The listing builds one solid part. Answer for the finished solid, in the listing's coordinates (mm). A direction names the side the tool comes from. Round coordinates to 2 decimals unless told otherwise and drop trailing zeros. Write each loop counter-clockwise with the first axis right and the second up, starting at its lowest first coordinate (ties: lowest second). Pieces come first, ordered by that corner, then holes.
(1) A cutting plane is placed at C-C, the plane y = 3.25. Give the vertices of the cut face in (x, z), and give its area (3 significant figures).
(2) Find the intervals of material crossed by probe 1 along X at (y, z) = (4.75, 23.5); probe 2 along Y at (x, z) = (2, -8.5); probe 3 along Y at (x, z) = (-14, -21.5), in increasing order.
(3) Each of these flat-tipped pins is pushed along its axis until it touches: pin 1 Ø1.2 at (y, z) = (4, -10) entering from -X; pin 2 Ø0.8 at (y, z) = (0.5, 26.5) entering from -X; pin 3 Ø3 at (y, z) = (4.5, -9) entering from -X; pin 4 Ø2 at (x, y) = (8.5, 1.5) entering from +Z. Where does it stop, or does it pass through?
(4) A cutting plane is placed at A-A, the plane x = 0. Give the vertices of the cut face in (y, z), and give its area (3 significant figures).
(5) A cutting plane is placed at D-D, the plane z = -15.5. Give the vertices of the cut face in (x, y).
(6) For faces 1 (the face through (5, 1, 1)), 2 (the face through (-12, 4, 1)), 3 (the face through (0.1, 0.5, 17.5)), determine the directions among +Z, -Z, +X, -X, +Y, -Y from which every point of the face is accessible in a straight line to the end or side of a thin tool.
(7) The mould has two halves that part along X. Classify faces 4 (the face through (12, 4, 1)), 5 (the face through (4, 0, 1)), 6 (the face through (0.1, 0.5, -17.5)): +X half, -X half, draft (parallel to the pull), parting line (faces both ways), or undercut.
(8) A cutting plane is placed at B-B, the plane z = -27.5. Give the vertices of the cut face in (x, y), and give its area (3 significant figures).
from build123d import *

# Parameters (mm, degrees)
BASE_EXTRUDE_THIN_DEPTH = 254
FILLET1_R               = 0.8
FILLET2_R               = 1.8
CUT_EXTRUDE1_DEPTH      = 255.685099682
LPATTERN1_COUNT         = 10
LPATTERN1_PITCH         = 25
MIRROR1_COPY_1_DEPTH    = 255.685099682
MIRROR1_COPY_2_DEPTH    = 255.685099682
MIRROR1_COPY_3_DEPTH    = 255.685099682
MIRROR1_COPY_4_DEPTH    = 255.685099682
MIRROR1_COPY_5_DEPTH    = 255.685099682
MIRROR1_COPY_6_DEPTH    = 255.685099682
MIRROR1_COPY_7_DEPTH    = 255.685099682
MIRROR1_COPY_8_DEPTH    = 255.685099682
MIRROR1_COPY_9_DEPTH    = 255.685099682
MIRROR1_COPY_10_DEPTH   = 255.685099682
SKETCH3_OUTSIDE_W       = 138.852
SKETCH3_OUTSIDE_H       = 611.852
SKETCH3_OUTSIDE_W_2     = 99.454563768
SKETCH3_OUTSIDE_H_2     = 76.2
CUT_EXTRUDE2_3_DEPTH    = 255.712583121


with BuildPart() as part:
    # Sketch1 → Base-Extrude-Thin (new, symmetric)
    with BuildSketch(Plane.XY):
        Polygon((-17.5, 6.5), (-12, 6.5), (-12, 0), (12, 0), (12, 6.5), (17.5, 6.5), (17.5, 7.5), (11, 7.5), (11, 1), (-11, 1), (-11, 7.5), (-17.5, 7.5), align=None)
    extrude(amount=BASE_EXTRUDE_THIN_DEPTH, both=True)

    # Fillet1
    fillet1_edges = [part.edges().sort_by_distance(p)[0] for p in [
        (-11, 1, 0),
        (11, 1, 0),
        (12, 6.5, 0),
        (-12, 6.5, 0),
    ]]
    fillet(fillet1_edges, radius=FILLET1_R)

    # Fillet2
    fillet2_edges = [part.edges().sort_by_distance(p)[0] for p in [
        (-11, 7.5, 0),
        (11, 7.5, 0),
        (12, 0, 0),
        (-12, 0, 0),
    ]]
    fillet(fillet2_edges, radius=FILLET2_R)

    # Sketch2 → Cut-Extrude1 (cut, through all)
    with BuildSketch(Plane(origin=(0, 1, 0), x_dir=(-1, 0, 0), z_dir=(0, 1, 0))):
        with BuildLine():
            Line((3.1, 4.4), (3.1, -4.4))
            ThreePointArc((3.1, -4.4), (0, -7.5), (-3.1, -4.4))
            Line((-3.1, -4.4), (-3.1, 4.4))
            ThreePointArc((-3.1, 4.4), (0, 7.5), (3.1, 4.4))
        make_face()
    cut_extrude1 = extrude(amount=-CUT_EXTRUDE1_DEPTH, mode=Mode.SUBTRACT)

    # LPattern1: Cut-Extrude1 ×10
    with Locations(*[(0, 0, -i * LPATTERN1_PITCH) for i in range(1, LPATTERN1_COUNT)]):
        add(cut_extrude1, mode=Mode.SUBTRACT)

    # Mirror1 copy 1 sketch → Mirror1 copy 1 (cut, through all)
    with BuildSketch(Plane(origin=(0, 1, 25), x_dir=(-1, 0, 0), z_dir=(0, 1, 0))):
        with BuildLine():
            Line((3.1, -4.4), (3.1, 4.4))
            ThreePointArc((3.1, 4.4), (0, 7.5), (-3.1, 4.4))
            Line((-3.1, 4.4), (-3.1, -4.4))
            ThreePointArc((-3.1, -4.4), (0, -7.5), (3.1, -4.4))
        make_face()
    extrude(amount=-MIRROR1_COPY_1_DEPTH, mode=Mode.SUBTRACT)

    # Mirror1 copy 2 sketch → Mirror1 copy 2 (cut, through all)
    with BuildSketch(Plane(origin=(0, 1, 50), x_dir=(-1, 0, 0), z_dir=(0, 1, 0))):
        with BuildLine():
            Line((3.1, -4.4), (3.1, 4.4))
            ThreePointArc((3.1, 4.4), (0, 7.5), (-3.1, 4.4))
            Line((-3.1, 4.4), (-3.1, -4.4))
            ThreePointArc((-3.1, -4.4), (0, -7.5), (3.1, -4.4))
        make_face()
    extrude(amount=-MIRROR1_COPY_2_DEPTH, mode=Mode.SUBTRACT)

    # Mirror1 copy 3 sketch → Mirror1 copy 3 (cut, through all)
    with BuildSketch(Plane(origin=(0, 1, 75), x_dir=(-1, 0, 0), z_dir=(0, 1, 0))):
        with BuildLine():
            Line((3.1, -4.4), (3.1, 4.4))
            ThreePointArc((3.1, 4.4), (0, 7.5), (-3.1, 4.4))
            Line((-3.1, 4.4), (-3.1, -4.4))
            ThreePointArc((-3.1, -4.4), (0, -7.5), (3.1, -4.4))
        make_face()
    extrude(amount=-MIRROR1_COPY_3_DEPTH, mode=Mode.SUBTRACT)

    # Mirror1 copy 4 sketch → Mirror1 copy 4 (cut, through all)
    with BuildSketch(Plane(origin=(0, 1, 100), x_dir=(-1, 0, 0), z_dir=(0, 1, 0))):
        with BuildLine():
            Line((3.1, -4.4), (3.1, 4.4))
            ThreePointArc((3.1, 4.4), (0, 7.5), (-3.1, 4.4))
            Line((-3.1, 4.4), (-3.1, -4.4))
            ThreePointArc((-3.1, -4.4), (0, -7.5), (3.1, -4.4))
        make_face()
    extrude(amount=-MIRROR1_COPY_4_DEPTH, mode=Mode.SUBTRACT)

    # Mirror1 copy 5 sketch → Mirror1 copy 5 (cut, through all)
    with BuildSketch(Plane(origin=(0, 1, 125), x_dir=(-1, 0, 0), z_dir=(0, 1, 0))):
        with BuildLine():
            Line((3.1, -4.4), (3.1, 4.4))
            ThreePointArc((3.1, 4.4), (0, 7.5), (-3.1, 4.4))
            Line((-3.1, 4.4), (-3.1, -4.4))
            ThreePointArc((-3.1, -4.4), (0, -7.5), (3.1, -4.4))
        make_face()
    extrude(amount=-MIRROR1_COPY_5_DEPTH, mode=Mode.SUBTRACT)

    # Mirror1 copy 6 sketch → Mirror1 copy 6 (cut, through all)
    with BuildSketch(Plane(origin=(0, 1, 150), x_dir=(-1, 0, 0), z_dir=(0, 1, 0))):
        with BuildLine():
            Line((3.1, -4.4), (3.1, 4.4))
            ThreePointArc((3.1, 4.4), (0, 7.5), (-3.1, 4.4))
            Line((-3.1, 4.4), (-3.1, -4.4))
            ThreePointArc((-3.1, -4.4), (0, -7.5), (3.1, -4.4))
        make_face()
    extrude(amount=-MIRROR1_COPY_6_DEPTH, mode=Mode.SUBTRACT)

    # Mirror1 copy 7 sketch → Mirror1 copy 7 (cut, through all)
    with BuildSketch(Plane(origin=(0, 1, 175), x_dir=(-1, 0, 0), z_dir=(0, 1, 0))):
        with BuildLine():
            Line((3.1, -4.4), (3.1, 4.4))
            ThreePointArc((3.1, 4.4), (0, 7.5), (-3.1, 4.4))
            Line((-3.1, 4.4), (-3.1, -4.4))
            ThreePointArc((-3.1, -4.4), (0, -7.5), (3.1, -4.4))
        make_face()
    extrude(amount=-MIRROR1_COPY_7_DEPTH, mode=Mode.SUBTRACT)

    # Mirror1 copy 8 sketch → Mirror1 copy 8 (cut, through all)
    with BuildSketch(Plane(origin=(0, 1, 200), x_dir=(-1, 0, 0), z_dir=(0, 1, 0))):
        with BuildLine():
            Line((3.1, -4.4), (3.1, 4.4))
            ThreePointArc((3.1, 4.4), (0, 7.5), (-3.1, 4.4))
            Line((-3.1, 4.4), (-3.1, -4.4))
            ThreePointArc((-3.1, -4.4), (0, -7.5), (3.1, -4.4))
        make_face()
    extrude(amount=-MIRROR1_COPY_8_DEPTH, mode=Mode.SUBTRACT)

    # Mirror1 copy 9 sketch → Mirror1 copy 9 (cut, through all)
    with BuildSketch(Plane(origin=(0, 1, 225), x_dir=(-1, 0, 0), z_dir=(0, 1, 0))):
        with BuildLine():
            Line((3.1, -4.4), (3.1, 4.4))
            ThreePointArc((3.1, 4.4), (0, 7.5), (-3.1, 4.4))
            Line((-3.1, 4.4), (-3.1, -4.4))
            ThreePointArc((-3.1, -4.4), (0, -7.5), (3.1, -4.4))
        make_face()
    extrude(amount=-MIRROR1_COPY_9_DEPTH, mode=Mode.SUBTRACT)

    # Mirror1 copy 10 sketch → Mirror1 copy 10 (cut, through all)
    with BuildSketch(Plane(origin=(0, 1, 0), x_dir=(-1, 0, 0), z_dir=(0, 1, 0))):
        with BuildLine():
            Line((3.1, -4.4), (3.1, 4.4))
            ThreePointArc((3.1, 4.4), (0, 7.5), (-3.1, 4.4))
            Line((-3.1, 4.4), (-3.1, -4.4))
            ThreePointArc((-3.1, -4.4), (0, -7.5), (3.1, -4.4))
        make_face()
    extrude(amount=-MIRROR1_COPY_10_DEPTH, mode=Mode.SUBTRACT)

    # Sketch3 outside → Cut-Extrude2 (3") (cut, through all)
    with BuildSketch(Plane(origin=(0, 7.5, 0), x_dir=(-1, 0, 0), z_dir=(0, 1, 0))):
        Rectangle(SKETCH3_OUTSIDE_W, SKETCH3_OUTSIDE_H)
        with Locations((-1.499324946, 0)):
            Rectangle(SKETCH3_OUTSIDE_W_2, SKETCH3_OUTSIDE_H_2, mode=Mode.SUBTRACT)
    extrude(amount=-CUT_EXTRUDE2_3_DEPTH, mode=Mode.SUBTRACT)


solid = part.part
Solutions:
1. outline: (-12, -38.1) - (-11, -38.1) - (-11, 38.1) - (-12, 38.1) - close; (11, -38.1) - (12, -38.1) - (12, 38.1) - (11, 38.1) - close
1. area: 152 mm2
2. probe 1: x = -12 to -11, 11 to 12
2. probe 2: y = 0 to 1
2. probe 3: y = 6.5 to 7.5
3. pin 1: stops at x = -12
3. pin 2: stops at x = -11.76
3. pin 3: stops at x = -12.06
3. pin 4: stops at z = 38.1
4. outline: (0, -38.1) - (1, -38.1) - (1, -32.5) - (0, -32.5) - close; (0, -17.5) - (1, -17.5) - (1, -7.5) - (0, -7.5) - close; (0, 7.5) - (1, 7.5) - (1, 17.5) - (0, 17.5) - close; (0, 32.5) - (1, 32.5) - (1, 38.1) - (0, 38.1) - close
4. area: 31.2 mm2
5. outline: (-17.5, 6.5) - (-12.8, 6.5) arc R0.8 cw to (-12, 5.7) - (-12, 1.8) arc R1.8 ccw to (-10.2, 0) - (10.2, 0) arc R1.8 ccw to (12, 1.8) - (12, 5.7) arc R0.8 cw to (12.8, 6.5) - (17.5, 6.5) - (17.5, 7.5) - (12.8, 7.5) arc R1.8 ccw to (11, 5.7) - (11, 1.8) arc R0.8 cw to (10.2, 1) - (-10.2, 1) arc R0.8 cw to (-11, 1.8) - (-11, 5.7) arc R1.8 ccw to (-12.8, 7.5) - (-17.5, 7.5) - close
6. face 1: +Z, -Z, +Y
6. face 2: +Z, -Z, -X, -Y
6. face 3: +Y, -Y
7. face 4: +X half
7. face 5: draft
7. face 6: undercut
8. outline: (-17.5, 6.5) - (-12.8, 6.5) arc R0.8 cw to (-12, 5.7) - (-12, 1.8) arc R1.8 ccw to (-10.2, 0) - (-3.1, 0) - (-3.1, 1) - (-10.2, 1) arc R0.8 cw to (-11, 1.8) - (-11, 5.7) arc R1.8 ccw to (-12.8, 7.5) - (-17.5, 7.5) - close; (3.1, 0) - (10.2, 0) arc R1.8 ccw to (12, 1.8) - (12, 5.7) arc R0.8 cw to (12.8, 6.5) - (17.5, 6.5) - (17.5, 7.5) - (12.8, 7.5) arc R1.8 ccw to (11, 5.7) - (11, 1.8) arc R0.8 cw to (10.2, 1) - (3.1, 1) - close
8. area: 39.6 mm2
